Verification items for the finished model (mm, model axes). A direction names the side the tool comes from. Round coordinates to 2 decimals unless told otherwise and drop trailing zeros. Write each loop counter-clockwise with the first axis right and the second up, starting at its lowest first coordinate (ties: lowest second). Pieces come first, ordered by that corner, then holes. Notation, with made-up numbers: (80.5, 66.25) - (120.5, 66.25) arc R12 cw to (120.5, 83.25) - close; hole circle Ø5 at (10, 57). An arc over 180 degrees is marked (long way). Answer as a JSON object with one key per item and string values. Group by question number.
1) Set-up check for faces 4 (the flat face through (72, 89, 2.8)), 5 (the cylindrical face through (66.07, 27, 1.38)): record each of +Z, -Z, +X, -X, +Y, -Y from which the full face is reachable in a straight line by a thin tool's end or side.
2) Thickness scan on line 1 (Y direction, x = 25.5, z = 1.45); line 2 (X direction, y = 143.5, z = 0.3); line 3 (Y direction, x = 68, z = 0.25). Record the ranges inside material, lowest first.
3) Section check B-B (x = 27). Enter the section's corners in (y, z), then the cut area to 3 significant figures.
4) Go/stop test with flat-tipped pins: pin 1 Ø6 at (x, y) = (67.5, 155) entering from +Z; pin 2 Ø0.6 at (y, z) = (81.5, 1) entering from -X. Record where each tip stops, or that it passes through.
5) Section check A-A (y = 155). Enter the section's corners in (x, z).
6) Section check D-D (y = 61). Enter the section's corners in (x, z).
7) Mould release check, pull along X, two halves, no side actions. Record for faces 1 (the cylindrical face through (66, 148.07, 1.38)), 2 (the flat face through (72, 89, 0)), 3 (the cylindrical face through (69, 22, 1)): +X half, -X half, draft (parallel to the pull), parting line (faces both ways), or undercut.
8) Section check C-C (z = 2.25). Enter the section's corners in (x, y).
```python
from build123d import *

# Parameters (mm, degrees)
F1_DEPTH = 2.8
F2_R     = 0.38
F3_DEPTH = 4
F4_R     = 2.5
F5_DEPTH = 2.801


with BuildPart() as f1:
    # F0 (on Top) → F1 (new body)
    with BuildSketch(Plane.XY):
        with BuildLine():
            Line((0, 25.5), (0, 0))
            Line((0, 0), (87.5, 0))
            Line((87.5, 0), (87.5, 175))
            Line((87.5, 175), (0, 175))
            Line((0, 175), (0, 149.5))
            Line((0, 149.5), (62.5, 149.5))
            ThreePointArc((62.5, 149.5), (66.035534, 148.035534), (67.5, 144.5))
            Line((67.5, 144.5), (67.5, 30.5))
            ThreePointArc((67.5, 30.5), (66.035534, 26.964466), (62.5, 25.5))
            Line((62.5, 25.5), (0, 25.5))
        make_face()
    extrude(amount=F1_DEPTH)

    # F2 (on face) → F3 (cut)
    with BuildSketch(Plane(origin=(67.5, 0, 0), x_dir=(0, -1, 0), z_dir=(-1, 0, 0))):
        with Locations((-106.55, 1.3)):
            Circle(F2_R)
        with Locations((-93.85, 1.3)):
            Circle(F2_R)
        with Locations((-81.15, 1.3)):
            Circle(F2_R)
        with Locations((-68.45, 1.3)):
            Circle(F2_R)
    extrude(amount=-F3_DEPTH, mode=Mode.SUBTRACT)

    # F4 (on face) → F5 (cut, through all)
    with BuildSketch(Plane.XY.offset(2.8)):
        with Locations((67.5, 155)):
            Circle(F4_R)
        with Locations((67.5, 20)):
            Circle(F4_R)
    extrude(amount=-F5_DEPTH, mode=Mode.SUBTRACT)


solid = f1.part
```
Returned:
{
 "1": {"face 4": "+Z, +X, -X, +Y, -Y", "face 5": "+Z, -Z, -X"},
 "2": {"line 1": "0 to 25.5, 149.5 to 175", "line 2": "67.5 to 87.5", "line 3": "0 to 17.55, 22.45 to 152.55, 157.45 to 175"},
 "3": {"outline": "(0, 0) - (25.5, 0) - (25.5, 2.8) - (0, 2.8) - close; (149.5, 0) - (175, 0) - (175, 2.8) - (149.5, 2.8) - close", "area": "143 mm2"},
 "4": {"pin 1": "z = 2.8", "pin 2": "x = 67.5"},
 "5": {"outline": "(0, 0) - (65, 0) - (65, 2.8) - (0, 2.8) - close; (70, 0) - (87.5, 0) - (87.5, 2.8) - (70, 2.8) - close"},
 "6": {"outline": "(67.5, 0) - (87.5, 0) - (87.5, 2.8) - (67.5, 2.8) - close"},
 "7": {"face 1": "-X half", "face 2": "draft", "face 3": "undercut"},
 "8": {"outline": "(0, 0) - (87.5, 0) - (87.5, 175) - (0, 175) - (0, 149.5) - (62.5, 149.5) arc R5 cw to (67.5, 144.5) - (67.5, 30.5) arc R5 cw to (62.5, 25.5) - (0, 25.5) - close; hole circle Ø5 at (67.5, 20); hole circle Ø5 at (67.5, 155)"}
}
